Input: dimensioned drawing with shaded views. Units: mm. Origin: part minimum x, y, z. A direction names the side the tool comes from. Round coordinates to 2 decimals unless told otherwise and drop trailing zeros. Loops run counter-clockwise (first coordinate to the right, second up) from the corner with the lowest first, then second, coordinate; pieces in that order, holes last. Notation, with made-up numbers: (17.25, -10) - (30.25, -10) arc R25 ccw to (30.25, 15) - close; hole circle Ø11 at (54.25, 77). An arc over 180 degrees is marked (long way). Answer as a JSON object with one key per item and string values. Group by question number.
Item 1: First-contact query: pin 1 (4 mm diameter, centred on x = 88.5, y = 44, fed in from +Z). Flat tip, straight axial feed; report the tip coordinate or a pass-through.
Item 2: Line query: line 1 (Z direction, x = 79, y = 41); line 2 (Y direction, x = 25.5, z = 145); line 3 (X direction, y = 51, z = 24.5). Output: solid intervals per line, ascending.
Item 3: Reachability of the marked faces 1, 2 and 3 from +Z, -Z, +X, -X, +Y, -Y: full face, straight path, thin tool, end or side. Return the list, or none.
Item 4: Section A-A (x = 38.5). Return the cut outline in (y, z), plus the area to 3 significant figures.
Item 5: Section B-B (y = 65.5). Return the cut outline in (x, z), plus the area to 3 significant figures.
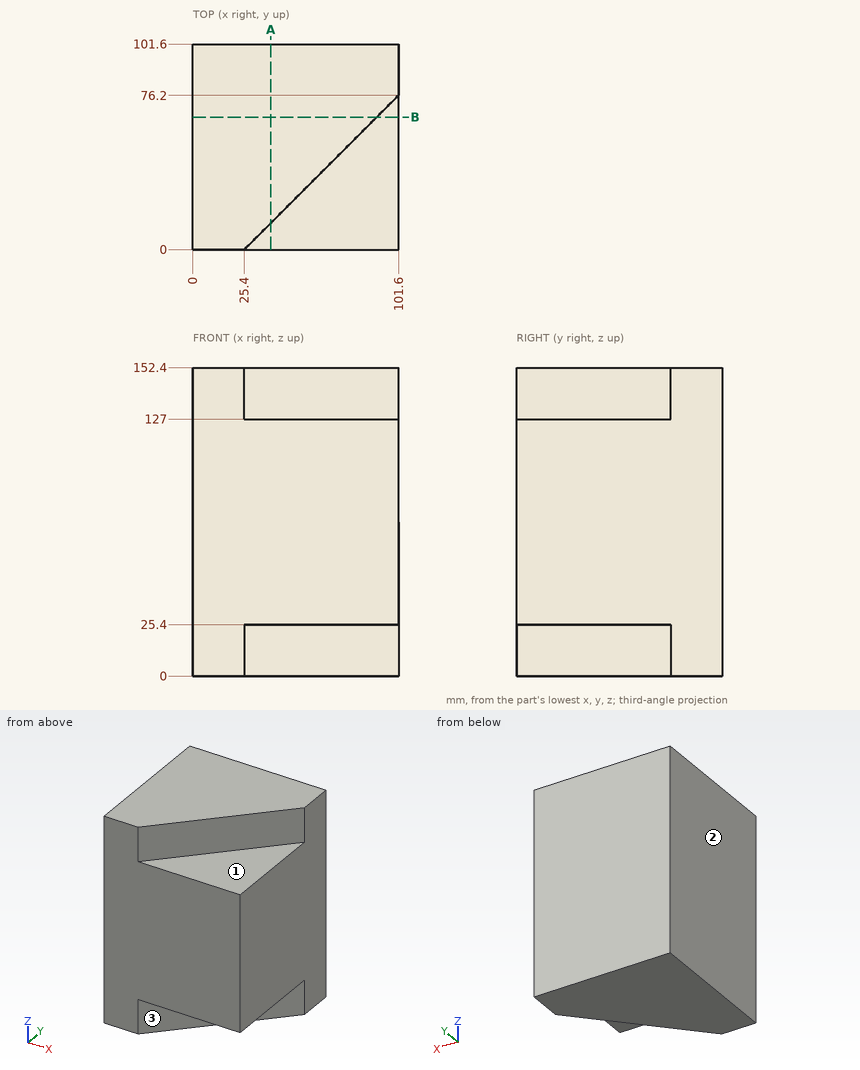
Values:
{
 "1": {"pin 1": "stops at z = 127"},
 "2": {"line 1": "z = 25.4 to 127", "line 2": "y = 0.1 to 101.6", "line 3": "x = 0 to 76.4"},
 "3": {"face 1": "+Z, +X, -Y", "face 2": "+Z, -Z, -X, +Y, -Y", "face 3": "-Z, +X, -Y"},
 "4": {"outline": "(0, 25.4) - (13.1, 25.4) - (13.1, 0) - (101.6, 0) - (101.6, 152.4) - (13.1, 152.4) - (13.1, 127) - (0, 127) - close", "area": "14,800 mm^2"},
 "5": {"outline": "(0, 0) - (90.9, 0) - (90.9, 25.4) - (101.6, 25.4) - (101.6, 127) - (90.9, 127) - (90.9, 152.4) - (0, 152.4) - close", "area": "14,900 mm^2"}
}
